The listing builds one solid part. Answer for the finished solid, in the listing's coordinates (mm). Round coordinates to 2 decimals unless told otherwise and drop trailing zeros. Write each loop counter-clockwise with the first axis right and the second up, starting at its lowest first coordinate (ties: lowest second). Pieces come first, ordered by that corner, then holes. Notation, with made-up numbers: (1.5, 10) - (36.5, 10) arc R26 ccw to (36.5, 44) - close; hole circle Ø9 at (6, -3). An arc over 180 degrees is marked (long way). Answer as CSV lines item,"result". Start each with the question number.
Item 1: Straight lines are drawn through the part: line 1 along Y through (x, z) = (-10, 6.5); line 2 along Y through (x, z) = (15, 7); line 3 along X through (y, z) = (10.5, 4). For each, find the intervals that lie inside material, in ascending order. Write a range as [from, to].
Item 2: A flat-ended cylindrical pin translates along its axis: pin 1 (1 mm diameter, centred on x = 12.5, z = 4, fed in from -Y). Find the tip coordinate at first contact, or state that the pin passes through.
Item 3: A cutting plane is placed at C-C on x = 15. State how many separate pieces and enclosed holes the cut face has, and give its area (3 significant figures).
Item 4: A cutting plane is placed at A-A on z = 1.5. Determine the outline of the cut face in (x, y).
Item 5: A cutting plane is placed at B-B on y = -9. Determine the outline of the cut face in (x, z).
```python
from build123d import *

# Parameters (mm, degrees)
SKETCH_1_W          = 40
SKETCH_1_H          = 40
EXTRUDE_1_DEPTH     = 10
SKETCH_2_R          = 1.6
CUT_EXTRUDE_1_DEPTH = 31
FILLET_1_R          = 10
FILLET_2_R          = 1


with BuildPart() as part:
    # 草图1 → 凸台-拉伸1 (new body)
    with BuildSketch(Plane.XY):
        Rectangle(SKETCH_1_W, SKETCH_1_H)
    extrude(amount=EXTRUDE_1_DEPTH)

    # 草图2 → 切除-拉伸1 (cut, through all)
    with BuildSketch(Plane.XY.offset(10)):
        with Locations((-10, 10)):
            Circle(SKETCH_2_R)
        with Locations(Location((15, 10, 0), (0, 0, 180))):
            Circle(SKETCH_2_R)
        with Locations((15, -10)):
            Circle(SKETCH_2_R)
        with Locations(Location((-10, -10, 0), (0, 0, 180))):
            Circle(SKETCH_2_R)
    extrude(amount=-CUT_EXTRUDE_1_DEPTH, mode=Mode.SUBTRACT)

    # 圆角1
    fillet_1_edges = [part.edges().sort_by_distance(p)[0] for p in [
        (20, -20, 5),
        (20, 20, 5),
    ]]
    fillet(fillet_1_edges, radius=FILLET_1_R)

    # 圆角2
    fillet_2_edges = [part.edges().sort_by_distance(p)[0] for p in [
        (-20, 0, 10),
        (-5, -20, 10),
        (20, 0, 0),
        (20, 0, 10),
        (-5, 20, 0),
        (17.071067812, 17.071067812, 0),
        (17.071067812, -17.071067812, 0),
        (-5, 20, 10),
        (17.071067812, 17.071067812, 10),
        (17.071067812, -17.071067812, 10),
        (-5, -20, 0),
        (-20, 0, 0),
        (-20, -20, 5),
        (-20, 20, 5),
    ]]
    fillet(fillet_2_edges, radius=FILLET_2_R)


solid = part.part
```
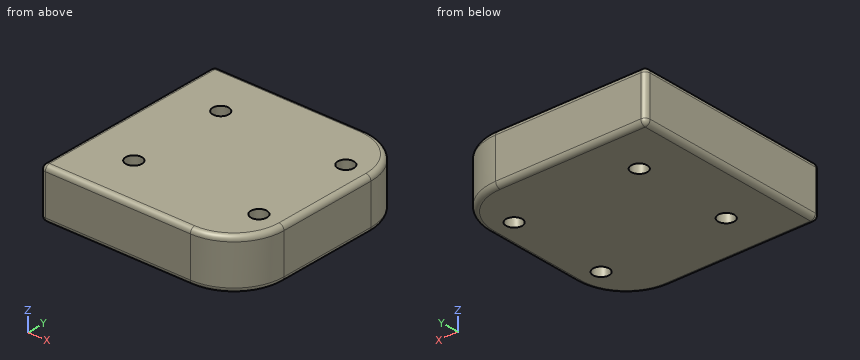
Geometry says:
1,line 1,"y = [-20, -11.6], [-8.4, 8.4], [11.6, 20]"
1,line 2,"y = [-18.66, -11.6], [-8.4, 8.4], [11.6, 18.66]"
1,line 3,"x = [-20, -11.52], [-8.48, 13.48], [16.52, 19.99]"
2,pin 1,"stops at y = -19.8"
3,separate pieces,"3"
3,enclosed holes,"0"
3,area,"308 mm^2"
4,outline,"(-20, -19) arc R1 ccw to (-19, -20) - (10, -20) arc R10 ccw to (20, -10) - (20, 10) arc R10 ccw to (10, 20) - (-19, 20) arc R1 ccw to (-20, 19) - close; hole circle Ø3.2 at (-10, -10); hole circle Ø3.2 at (-10, 10); hole circle Ø3.2 at (15, -10); hole circle Ø3.2 at (15, 10)"
5,outline,"(-20, 1) arc R1 ccw to (-19, 0) - (-11.25, 0) - (-11.25, 10) - (-19, 10) arc R1 ccw to (-20, 9) - close; (-8.75, 0) - (13.75, 0) - (13.75, 10) - (-8.75, 10) - close; (16.25, 0) - (19, 0) arc R1 ccw to (20, 1) - (20, 9) arc R1 ccw to (19, 10) - (16.25, 10) - close"
